from build123d import *

# Parameters (mm, degrees)
F1_DEPTH       = 250
F3_D           = 11
F3_CSINK_D     = 22.4
F3_CSINK_ANGLE = 90
F5_D           = 11


with BuildPart() as f1:
    # F0 (on Front) → F1 (new body, symmetric)
    with BuildSketch(Plane.XZ):
        Polygon((-541.7919028829, 43.9059940034), (-520.8959514415, 21.9529970017), (-515.1013105541, 27.4686236195), (-538.3620118087, 51.9059940034), (-581.7919028829, 51.9059940034), (-581.7919028829, 43.9059940034), align=None)
        Polygon((-500, 0), (0, 0), (0, 8), (-496.5701089258, 8), (-515.1013105541, 27.4686236195), (-520.8959514415, 21.9529970017), align=None)
    extrude(amount=F1_DEPTH, both=True)

    # F3 (through all)
    with Locations(Plane(origin=(0, 0, 0), x_dir=(1, 0, 0), z_dir=(0, 0, -1))):
        with Locations((-450, 200), (-50, 200), (-50, -200), (-450, -200)):
            CounterSinkHole(F3_D / 2, F3_CSINK_D / 2, counter_sink_angle=F3_CSINK_ANGLE)

    # F5 (through all)
    with Locations(Plane(origin=(0, 0, 43.9059940034), x_dir=(1, 0, 0), z_dir=(0, 0, -1))):
        with Locations((-561.7919028829, 190), (-561.7919028829, -190)):
            Hole(F5_D / 2)


solid = f1.part
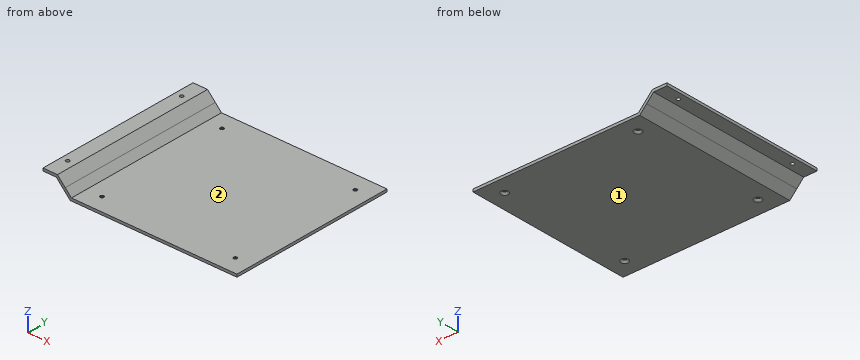
Here's how the part is built. I have some questions about the finished solid (model axes, mm). Face numbers are marked on the shaded views. A direction names the side the tool comes from. Round coordinates to 2 decimals unless told otherwise and drop trailing zeros. Order: outer loops, then holes, each group sorted by start corner. A loop starts at its lowest first (then second) coordinate and runs counter-clockwise, first axis right, second up. Notation, with made-up numbers: (25.5, -27) -> (33.5, -27) arc R6 cw to (33.5, -20) -> close; hole circle Ø9 at (-2.75, 75.5). An arc over 180 degrees is marked (long way). Use CSV: the item, a comma, the result in double quotes.
1. I want a section at A-A on y = 115.5. List the corners of the cut face in (x, z) for me.
Recorded:
outline,"(-581.79, 43.91) -> (-541.79, 43.91) -> (-500, 0) -> (0, 0) -> (0, 8) -> (-496.57, 8) -> (-538.36, 51.91) -> (-581.79, 51.91) -> close"
2. I want a section at B-B on x = -84. List the corners of the cut face in (y, z) for me, and give its area (3 significant figures).
Recorded:
outline,"(-250, 0) -> (250, 0) -> (250, 8) -> (-250, 8) -> close"
area,"4,000 mm2"
3. I need wall thicknesses on line 1 along Y through (x, z) = (-50, 6.5); line 2 along X through (y, z) = (-200, 7.05); line 3 along X through (y, z) = (-200, 6.9). Which ranges of each line are inside material? Lowest first, please.
Recorded:
line 1,"y = -250 to -205.5, -194.5 to 194.5, 205.5 to 250"
line 2,"x = -506.71 to -455.5, -444.5 to -55.5, -44.5 to 0"
line 3,"x = -506.57 to -455.5, -444.5 to -55.5, -44.5 to 0"
4. I'm going to push flat-ended pins straight in: P1, Ø9, axis at x = -450, y = -200, coming from the +Z side; P2, Ø17.5, axis at x = -561.79, y = -190, coming from the -Z side; P3, Ø1.5, axis at y = -17.5, z = 15, coming from the -X side; P4, Ø6, axis at y = 154, z = 41.5, coming from the -X side. Where does each tip first touch, or does it pass through?
Recorded:
P1,"passes through"
P2,"stops at z = 43.91"
P3,"stops at x = -514.99"
P4,"stops at x = -581.79"
5. Which directions (+Z, -Z, +X, -X, +Y, -Y) give clear straight access to the entire face, cutting with the end or side of a thin tool? Please do the marked faces 1 and 2.
Recorded:
face 1,"-Z, +X, -X, +Y, -Y"
face 2,"+Z, +X, +Y, -Y"
